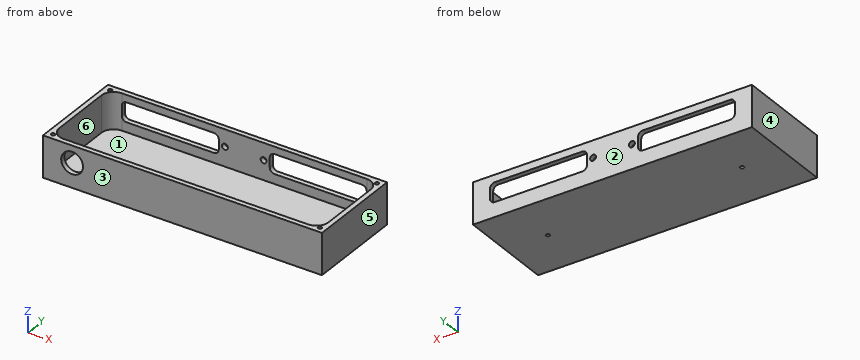
Autodesk Inventor part; units mm, degrees
ref_plane "YZ Plane" through (0, 0, 0) normal (1, 0, 0) x (0, 1, 0)
ref_plane "XZ Plane" through (0, 0, 0) normal (0, 1, 0) x (-1, 0, 0)
ref_plane "XY Plane" through (0, 0, 0) normal (0, 0, 1) x (1, 0, 0)
sketch "Skizze1" plane through (0, 0, 0) normal (0, 0, 1) x (1, 0, 0)
  line L0 (-23, 0) -> (138, 0)
  line L1 (0, -8) -> (0, 48)
  line L2 (0, 0) -> (115, 0)
  line L3 (115, 0) -> (115, 40)
  line L4 (115, 40) -> (0, 40)
  line L5 (0, 40) -> (0, 0)
  dimension "d0" = 40
  dimension "d1" = 115
extrude "Extrusion1" add sketch "Skizze1" along normal blind 17
sketch "Skizze2" plane through (0, 0, 17) normal (0, 0, 1) x (1, 0, 0)
  line L0 (0, 0) -> (115, 0)
  line L1 (115, 0) -> (115, 40)
  line L2 (115, 40) -> (0, 40)
  line L3 (0, 40) -> (0, 0)
  line L4 (7, 38) -> (108, 38)
  line L5 (113, 33) -> (113, 7)
  line L6 (108, 2) -> (7, 2)
  line L7 (2, 7) -> (2, 33)
  arc A0 (7, 38) -> (2, 33) centre (7, 33) ccw
  arc A1 (113, 33) -> (108, 38) centre (108, 33) ccw
  arc A2 (108, 2) -> (113, 7) centre (108, 7) ccw
  arc A3 (2, 7) -> (7, 2) centre (7, 7) ccw
  dimension "d4" = 2
  dimension "d5" = 5
extrude "Extrusion2" cut sketch "Skizze2" against normal blind 15 contours L4 A1 L5 A2 L6 A3 L7 A0
sketch "Skizze3" plane through (0, 0, 17) normal (0, 0, 1) x (1, 0, 0)
  line L0 (0, 0) -> (115, 0)
  line L1 (115, 0) -> (115, 40)
  line L2 (115, 40) -> (0, 40)
  line L3 (0, 40) -> (0, 0)
  line L4 (2.5, 37.5) -> (112.5, 37.5)
  line L5 (112.5, 37.5) -> (112.5, 2.5)
  line L6 (112.5, 2.5) -> (2.5, 2.5)
  line L7 (2.5, 2.5) -> (2.5, 37.5)
  dimension "d8" = 2.5
hole "Bohrung1" at (112.5, 37.5, 17) at (112.5, 2.5, 17) at (2.5, 2.5, 17) at (2.5, 37.5, 17) direction (0, 0, -1) diameter 1.567 depth 6 tip angle 118
sketch "Skizze4" plane through (0, 40, 0) normal (0, 1, 0) x (1, 0, 0)
  line L0 (0, 0) -> (0, -17)
  line L1 (113, -17) -> (108, -17)
  line L2 (113, -17) -> (108, -17)
  line L3 (113, -17) -> (113, -2)
  line L4 (113, -2) -> (108, -2)
  line L5 (108, -17) -> (108, -2)
  line L6 (108, -17) -> (7, -17)
  line L7 (108, -17) -> (108, -2)
  line L8 (108, -2) -> (7, -2)
  line L9 (7, -17) -> (7, -2)
  line L10 (88, -11) -> (88, -16)
  line L11 (108, -11) -> (88, -11)
  line L12 (108, -16) -> (108, -11)
  line L13 (88, -16) -> (108, -16)
  line L14 (-60.4, 0) -> (362.4, 0)
  line L15 (0, 3.4) -> (0, -20.4)
  arc A0 (118, -8) -> (118, -12) centre (118, -10) ccw
  line L16 (302, -14) -> (294, -14)
  line L17 (302, -6) -> (302, -14)
  line L18 (294, -6) -> (302, -6)
  line L19 (106, -14) -> (70, -14)
  line L20 (68, -12) -> (68, -8)
  line L21 (70, -6) -> (106, -6)
  line L22 (108, -8) -> (108, -12)
  arc A1 (108, -8) -> (106, -6) centre (106, -8) ccw
  arc A2 (106, -14) -> (108, -12) centre (106, -12) ccw
  arc A3 (68, -12) -> (70, -14) centre (70, -12) ccw
  arc A4 (70, -6) -> (68, -8) centre (70, -8) ccw
  line L23 (45, -14) -> (9, -14)
  line L24 (7, -12) -> (7, -8)
  line L25 (9, -6) -> (45, -6)
  line L26 (47, -8) -> (47, -12)
  arc A5 (45, -14) -> (47, -12) centre (45, -12) ccw
  arc A6 (47, -8) -> (45, -6) centre (45, -8) ccw
  arc A7 (9, -6) -> (7, -8) centre (9, -8) ccw
  arc A8 (7, -12) -> (9, -14) centre (9, -12) ccw
  line L27 (115, 0) -> (115, -17)
  arc A9 (283, -8) -> (281, -6) centre (281, -8) ccw
  line L28 (283, -8) -> (283, -12)
  arc A10 (281, -14) -> (283, -12) centre (281, -12) ccw
  line L29 (294, -14) -> (281, -14)
  line L30 (281, -6) -> (294, -6)
  point P0 (6, -6)
  point P1 (6, -14)
  point P2 (108, -14)
  point P3 (68, -6)
  point P4 (68, -14)
  point P5 (47, -14)
  point P6 (7, -6)
  dimension "d16" = 40
  dimension "d17" = 2
  dimension "d18" = 7
  dimension "d19" = 40
  dimension "d20" = 2
  dimension "d23" = 7
extrude "Extrusion3" cut sketch "Skizze4" against normal blind 2 contours A2 L19 L10 L11 L5 | L9 A7 L25 A6 L26 A5 L23 A8 | L5 L11 L10 L19 A3 L20 A4 L21 A1
sketch "Skizze5" plane through (0, 40, 0) normal (0, 1, 0) x (1, 0, 0)
  line L0 (0, 0) -> (0, -17)
  line L1 (115, -17) -> (0, -17)
  line L2 (115, 0) -> (115, -17)
  line L3 (0, -10) -> (115, -10)
  line L4 (115, 0) -> (0, 0)
  line L5 (57.5, -10) -> (57.5, -13.4142)
  point P0 (49.5, -10)
  point P1 (65.5, -10)
  dimension "d24" = 7
  dimension "d35" = 16
hole "Bohrung2" at (49.5, 40, 10) at (65.5, 40, 10) direction (0, -1, 0) diameter 2.459 depth 8 tip angle 118
sketch "Skizze6" plane through (0, 0, 2) normal (0, 0, 1) x (1, 0, 0)
  line L0 (7, 38) -> (108, 38)
  line L1 (2, 7) -> (2, 33)
  line L2 (113, 33) -> (113, 7)
  line L3 (-23, 0) -> (138, 0)
  line L4 (0, -8) -> (0, 48)
  line L5 (2, 20) -> (113, 20)
  line L6 (57.5, 38) -> (57.5, 39.5212)
  point P0 (0, 0)
  point P1 (17.5, 20)
  point P2 (97.5, 20)
  dimension "d36" = 80
hole "Bohrung3" at (17.5, 20, 2) at (97.5, 20, 2) direction (0, 0, -1) diameter 1.567 end through all
sketch "Skizze7" plane through (0, 0, 0) normal (0, -1, 0) x (1, 0, 0)
  line L0 (0, 0) -> (115, 0)
  line L1 (0, 0) -> (0, 17)
  line L2 (0, 10) -> (20.9799, 10)
  line L3 (7, 17) -> (7, 2)
  point P0 (12, 10)
  dimension "d44" = 10
  dimension "d45" = 12
hole "Bohrung4" at (12, 0, 10) direction (0, 1, 0) diameter 9 end up to surface
properties part number "13_1087_023"
CAD build for the part. Positions are in the model's coordinates, mm. Face numbers are marked on the shaded views. A direction names the side the tool comes from. Coordinates: 2 decimals unless noted, no trailing zeros. Loops run counter-clockwise (first coordinate to the right, second up) from the corner with the lowest first, then second, coordinate; pieces in that order, holes last. Notation, with made-up numbers: (-36.5, -12.75) - (-14.5, -12.75) arc R19 ccw to (-14.5, 10.25) - close; hole circle Ø5 at (36, 19.25). An arc over 180 degrees is marked (long way). Return JSON: item names as keys, results as strings.
1. Band-saw the part on D-D (y = 24.5). Give the cut face in (x, z).
Result:
{"outline": "(0, 0) - (115, 0) - (115, 17) - (113, 17) - (113, 2) - (2, 2) - (2, 17) - (0, 17) - close"}
2. Probe L1, parallel to X at y = 38.7, z = 10; L2, parallel to X at y = 2.5, z = 15.15; L3, parallel to X at y = 10, z = 3. List the from-to ranges inside material, lowest first. Write a range as from..to.
Result:
{"L1": "x = 0..7, 47..48.27, 50.73..64.27, 66.73..68, 108..115", "L2": "x = 0..1.72, 3.28..4.82, 110.18..111.72, 113.28..115", "L3": "x = 0..2, 113..115"}
3. Drop flat-ended pins along their axis: pin 1 (0.9 mm diameter, centred on x = 17.5, y = 20, fed in from -Z); pin 2 (2 mm diameter, centred on x = 97.5, y = 20, fed in from +Z). Give the stop position or say it passes through.
Result:
{"pin 1": "passes through", "pin 2": "stops at z = 2"}
4. Band-saw the part on B-B (x = 12). Give the cut face in (y, z).
Result:
{"outline": "(0, 0) - (40, 0) - (40, 6) - (38, 6) - (38, 2) - (2, 2) - (2, 5.5) - (0, 5.5) - close; (0, 14.5) - (2, 14.5) - (2, 17) - (0, 17) - close; (38, 14) - (40, 14) - (40, 17) - (38, 17) - close"}
5. 3-axis set-ups, long thin cutter, end or side, ignore diameter. For the marked faces 1 and 2: which of +Z, -Z, +X, -X, +Y, -Y reach the whole face in a straight line?
Result:
{"face 1": "+Z", "face 2": "+Z, -Z, +X, -X, +Y"}
6. Band-saw the part on A-A (x = 65.5). Give the cut face in (y, z).
Result:
{"outline": "(0, 0) - (40, 0) - (40, 8.77) - (38, 8.77) - (38, 2) - (2, 2) - (2, 17) - (0, 17) - close; (38, 11.23) - (40, 11.23) - (40, 17) - (38, 17) - close"}
7. Mould opens along X. For the marked faces 3, 4, 5 and 6 say: released by +X, released by -X, zero draft, split by the parting line, or undercut.
Result:
{"face 3": "zero draft", "face 4": "released by -X", "face 5": "released by +X", "face 6": "undercut"}
8. Band-saw the part on C-C (z = 15.75). Give the cut face in (x, y), and give its area (3 significant figures).
Result:
{"outline": "(0, 0) - (115, 0) - (115, 40) - (0, 40) - close; hole circle Ø1.57 at (2.5, 2.5); hole circle Ø1.57 at (2.5, 37.5); hole (2, 7) arc R5 ccw to (7, 2) - (108, 2) arc R5 ccw to (113, 7) - (113, 33) arc R5 ccw to (108, 38) - (7, 38) arc R5 ccw to (2, 33) - close; hole circle Ø1.57 at (112.5, 2.5); hole circle Ø1.57 at (112.5, 37.5)", "area": "618 mm2"}
